Work out the finished part from the listing and answer in its coordinate system (mm). A direction names the side the tool comes from. Coordinates: 2 decimals unless noted, no trailing zeros. Loops run counter-clockwise (first coordinate to the right, second up) from the corner with the lowest first, then second, coordinate; pieces in that order, holes last. Notation, with made-up numbers: M 25.5,61.5 L 81.5,61.5 A5 cw 81.5,65.5 Z; hole C -36,32.25 d11. An arc over 180 degrees is marked long. Write each question's results on one line, items separated by ' | '.
Autodesk Inventor part; units mm, degrees
ref_plane "Work Plane2" through (0, 3, 0) normal (0, 1, 0) x (1, 0, 0)
ref_plane "YZ Plane" through (0, 0, 0) normal (1, 0, 0) x (0, 1, 0)
ref_plane "XZ Plane" through (0, 0, 0) normal (0, 1, 0) x (-1, 0, 0)
sketch "Sketch1" plane through (0, 0, 0) normal (0, 1, 0) x (-1, 0, 0)
  line L0 (0, 0) -> (-30, 0)
  line L1 (-30, 0) -> (-20, -70)
  line L2 (-20, -70) -> (-10, -70)
  line L3 (-10, -70) -> (0, 0)
  line L4 (-30, 0) -> (-20, 80)
  line L5 (-20, 80) -> (-10, 80)
  line L6 (-10, 80) -> (0, 0)
  line L7 (-21.6955, 10) -> (-8.3045, 10)
  line L8 (-8.3045, 10) -> (-15, 63.5642)
  line L9 (-15, 63.5642) -> (-21.6955, 10)
  line L10 (-21.5004, -10) -> (-8.4996, -10)
  line L11 (-8.4996, -10) -> (-15, -55.5025)
  line L12 (-15, -55.5025) -> (-21.5004, -10)
  dimension "d15" = 80
  dimension "d16" = 70
  dimension "d17" = 10
  dimension "d18" = 10
  dimension "d19" = 30
  dimension "d20" = 10
  dimension "d21" = 10
  dimension "d40" = 10
  dimension "d41" = 10
  dimension "d42" = 7
  dimension "d43" = 7
  dimension "d45" = 7
  dimension "d46" = 7
ref_plane "Work Plane2" through (0, 3, 0) normal (0, 1, 0) x (1, 0, 0)
sketch "Sketch3" plane through (0, 3, 0) normal (0, 1, 0) x (1, 0, 0)
  line L0 (29.1194, -1.55) -> (0.2583, -1.55)
  line L1 (0.5917, -3.55) -> (0.2583, -1.55)
  line L2 (0.5917, -3.55) -> (29.4083, -3.55)
  line L3 (29.69, 1.55) -> (29.29, 3.55)
  line L4 (29.29, 3.55) -> (0.71, 3.55)
  line L5 (0.71, 3.55) -> (0.31, 1.55)
  line L6 (0.31, 1.55) -> (29.69, 1.55)
  line L7 (30, 0) -> (0, 0)
  line L8 (29.4083, -3.55) -> (29.7417, -1.55)
  line L9 (29.1194, -1.55) -> (29.7417, -1.55)
  line L10 (20, 50) -> (10, 50)
  line L11 (20, -60) -> (10, -60)
  line L12 (30, 0) -> (20, 50)
  line L13 (10, -60) -> (0, 0)
  line L14 (30, 0) -> (20, -60)
  line L15 (10, 50) -> (0, 0)
  dimension "d26" = 1.55
  dimension "d27" = 1.55
  dimension "d28" = 2
  dimension "d29" = 2
extrude "Extrusion5" add sketch "Sketch1" along normal blind 4
fillet "Fillet3" radius 5.75 4 edges at (20, 2, 80) (10, 2, 80) (20, 2, -70) (10, 2, -70)
fillet "Fillet4" radius 0.5 2 edges at (15, 2, 63.5642) (15, 2, -55.5025)
extrude "Extrusion7" add sketch "Sketch3" along normal blind 30 contours L9 L8 L2 L1 L0 | L5 L4 L3 L6
fillet "Fillet5" radius 6.45 2 edges at (15, 4, -3.55) (15, 4, 3.55)
equation "\"d18\" = d17"
equation "\"d20\" = d17"
equation "\"d21\" = d17"
equation "\"d43\" = d42"
equation "\"d45\" = d42"
equation "\"d46\" = d42"
equation "\"d27\" = d26"
equation "\"d29\" = d28"
properties part number "support"
1) Find section D-D, the plane x = 13. Give the number of separate pieces and of enclosed holes in the cut face, and give its area (3 significant figures).
Check result:
separate pieces: 3 | enclosed holes: 0 | area: 452 mm^2
2) Which of the six approach directions +Z, -Z, +X, -X, +Y, -Y give full straight-line access (tool end or side, diameter ignored) to faces 4 (the face through (0.5, 16.3, 3)), 5 (the face through (29.41, 16.28, -2.94)), 6 (the face through (15, 2, -10))?
Check result:
face 4: +Z, -X, +Y | face 5: -Z, +X, +Y | face 6: +Y, -Y
3) For a pull along Z with two mould halves and no side action, classify faces 1 (the face through (29.5, 16.3, 3)), 2 (the face through (0.6, 16.3, -3)), 3 (the face through (18.456, 1.972, -31.313)) as released by +Z, released by -Z, zero draft, split by the parting line, or undercut.
Check result:
face 1: released by +Z | face 2: released by -Z | face 3: undercut
4) Find section B-B, the plane z = 54. Give the vertices of the cut face in (x, y), and give its area (3 significant figures).
Check result:
outline: M 6.75,0 L 13.8,0 L 13.8,4 L 6.75,4 Z; M 16.2,0 L 23.25,0 L 23.25,4 L 16.2,4 Z | area: 56.4 mm^2
5) Straight lines are drawn through the part: probe 1 along Z at (x, y) = (6, 19); probe 2 along Y at (x, z) = (18, -55.5); probe 3 along X at (y, z) = (3.5, -49.5). For each, find the intervals that lie inside material, in ascending order. Write a range as [from, to].
Check result:
probe 1: [-3.55, -1.55], [1.55, 3.55] | probe 2: [0, 4] | probe 3: [7.07, 14.14], [15.86, 22.93]
6) Find section A-A, the plane y = 13. Give the vertices of the cut face in (x, z), and give its area (3 significant figures).
Check result:
outline: M 0.26,1.55 L 29.74,1.55 L 29.41,3.55 L 0.59,3.55 Z; M 0.31,-1.55 L 0.71,-3.55 L 29.29,-3.55 L 29.69,-1.55 Z | area: 116 mm^2
7) Given pin 1 Ø1 at (y, z) = (13.5, 6) entering from +X; pin 2 Ø10 at (x, z) = (12.5, -5.5) entering from +Y; pin 3 Ø10 at (x, y) = (11, 18.5) entering from -Z; pin 4 Ø4 at (x, z) = (13, 47) entering from +Y, each flat-ended and moving along its own axis, determine where each tip first touches the part or whether it passes through.
Check result:
pin 1: through | pin 2: y = 33 | pin 3: z = -3.55 | pin 4: y = 4
8) Find section C-C, the plane x = 7. Give the vertices of the cut face in (y, z).
Check result:
outline: M 0,-49 L 4,-49 L 4,-10 A6.45 cw 10.45,-3.55 L 33,-3.55 L 33,-1.55 L 4,-1.55 L 4,1.55 L 33,1.55 L 33,3.55 L 10.45,3.55 A6.45 cw 4,10 L 4,56 L 0,56 Z
